For this review, take the finished solid that the model builds, in its own axes (mm). A direction names the side the tool comes from. Round coordinates to 2 decimals unless told otherwise and drop trailing zeros. Order: outer loops, then holes, each group sorted by start corner. A loop starts at its lowest first (then second) coordinate and runs counter-clockwise, first axis right, second up.
from build123d import *

# Parameters (mm, degrees)
F1_DEPTH = 25.4


with BuildPart() as f1:
    # F0 (on Front) → F1 (new body)
    with BuildSketch(Plane.XZ):
        with BuildLine():
            Line((-59.0061545372, 19.8315382004), (-59.0061545372, 0))
            Line((-59.0061545372, 0), (-57.6384626329, 0))
            Line((-57.6384626329, 0), (-52.8619785953, 0))
            ThreePointArc((-52.8619785953, 0), (-52.785725887, 1.0863777847), (-52.5584630668, 2.1514518559))
            Line((-52.5584630668, 2.1514518559), (-52.5584630668, 5.3730774671))
            Line((-52.5584630668, 5.3730774671), (-48.7484624609, 9.183078073))
            Line((-48.7484624609, 9.183078073), (-41.4215400815, 9.183078073))
            Line((-41.4215400815, 9.183078073), (-37.6115394756, 5.3730774671))
            Line((-37.6115394756, 5.3730774671), (-37.6115394756, 4.7639395972))
            ThreePointArc((-37.6115394756, 4.7639395972), (-38.2208958426, 4.7248074356), (-38.8202414059, 4.6080538331))
            ThreePointArc((-38.8202414059, 4.6080538331), (-37.6957431315, 2.4249207086), (-37.3080239472, 0))
            Line((-37.3080239472, 0), (23.1979270853, 0))
            ThreePointArc((23.1979270853, 0), (23.2602248919, 1.000404867), (23.446155712, 1.9853518934))
            ThreePointArc((23.446155712, 1.9853518934), (30.0178470159, 7.9671258273), (38.0999986082, 4.2728638401))
            ThreePointArc((38.0999986082, 4.2728638401), (39.0128166681, 2.2225195794), (39.3251548134, 0))
            Line((39.3251548134, 0), (48.2600033283, 0))
            Line((48.2600033283, 0), (48.2600033283, 16.9007703662))
            Line((48.2600033283, 16.9007703662), (48.2600033283, 19.8315382004))
            Line((48.2600033283, 19.8315382004), (47.6738475263, 22.3715398461))
            Line((47.6738475263, 22.3715398461), (25.399999693, 22.3715398461))
            Line((25.399999693, 22.3715398461), (12.1138468385, 35.6576927006))
            Line((12.1138468385, 35.6576927006), (-28.3307693899, 35.6576927006))
            Line((-28.3307693899, 35.6576927006), (-28.3307693899, 19.8315382004))
            Line((-28.3307693899, 19.8315382004), (-59.0061545372, 19.8315382004))
        make_face()
        with BuildLine():
            ThreePointArc((-52.5584630668, 2.1514518559), (-52.785725887, 1.0863777847), (-52.8619785953, 0))
            Line((-52.8619785953, 0), (-52.5584630668, 0))
            Line((-52.5584630668, 0), (-52.5584630668, 2.1514518559))
        make_face()
        with BuildLine():
            Line((-52.5584630668, 0), (-52.8619785953, 0))
            ThreePointArc((-52.8619785953, 0), (-45.0850012712, -7.776977324), (-37.3080239472, 0))
            ThreePointArc((-37.3080239472, 0), (-37.6957431315, 2.4249207086), (-38.8202414059, 4.6080538331))
            ThreePointArc((-38.8202414059, 4.6080538331), (-46.4539291026, 7.6555478505), (-52.5584630668, 2.1514518559))
            Line((-52.5584630668, 2.1514518559), (-52.5584630668, 0))
        make_face()
        with BuildLine():
            Line((23.446155712, 0), (23.1979270853, 0))
            ThreePointArc((23.1979270853, 0), (31.2615409493, -8.0636138641), (39.3251548134, 0))
            Line((39.3251548134, 0), (38.0999986082, 0))
            Line((38.0999986082, 0), (23.446155712, 0))
        make_face()
        with BuildLine():
            ThreePointArc((23.446155712, 1.9853518934), (23.2602248919, 1.000404867), (23.1979270853, 0))
            Line((23.1979270853, 0), (23.446155712, 0))
            Line((23.446155712, 0), (23.446155712, 1.9853518934))
        make_face()
        with BuildLine():
            Line((38.0999986082, 0), (39.3251548134, 0))
            ThreePointArc((39.3251548134, 0), (39.0128166681, 2.2225195794), (38.0999986082, 4.2728638401))
            Line((38.0999986082, 4.2728638401), (38.0999986082, 0))
        make_face()
        with BuildLine():
            ThreePointArc((38.0999986082, 4.2728638401), (30.0178470159, 7.9671258273), (23.446155712, 1.9853518934))
            Line((23.446155712, 1.9853518934), (23.446155712, 0))
            Line((23.446155712, 0), (38.0999986082, 0))
            Line((38.0999986082, 0), (38.0999986082, 4.2728638401))
        make_face()
    extrude(amount=F1_DEPTH)


solid = f1.part
(1) Add section A-A on y = -23. Give the boundary of the cut face in (x, z) (3 decimals).
(2) Wall thickness on L1, parallel to X at y = -18.75, z = 6; L2, parallel to X at y = -21.75, z = -0.5; L3, parallel to X at y = -1.5, z = -6: over which ranges is each line inside the solid? List them lowest first.
(3) Draft analysis for pull direction Z (two halves, no side actions). For faces 6 (the face through (-28.331, -13, 28)), 7 (the face through (-50.68, -12.52, 7.25)), 8 (the face through (-8, -13, 35.658)), 9 (the face through (-46.334, -12.522, 7.676)), state which applies: pulls with the +Z half, pulls with the -Z half, needs draft (parallel to the pull), parting line crosses it, or undercut.
(4) Add section C-C on z = 30. Give the boundary of the cut face in (x, y), plus the area to 3 significant figures.
(5) Add section B-B on x = -33. Give the boundary of the cut face in (y, z).
(6) Tool access review of faces 1 (the face through (44, -13, 0)), 2 (the face through (37, -13, 22.372)), 3 (the face through (-56, -13, 0)), 4 (the face through (-7, -13, 0)), 5 (the face through (-45, -13, 9.183)): name each direction out of +Z, -Z, +X, -X, +Y, -Y from which nothing blocks a thin tool from reaching the whole face with its end or side.
(7) Clearance check with flat-ended pins moving along their axes: P1, Ø7, axis at x = -57, y = -12, coming from the -Z side; P2, Ø6, axis at y = -12.5, z = 26.5, coming from the +X side; P3, Ø8, axis at x = 24, y = -15.5, coming from the +Z side. State where each tip first meets the part, or that it passes through.
Here are the results:
1. outline: (-59.006, 0) - (-52.862, 0) arc R7.777 ccw to (-37.308, 0) - (23.198, 0) arc R8.064 ccw to (39.325, 0) - (48.26, 0) - (48.26, 19.832) - (47.674, 22.372) - (25.4, 22.372) - (12.114, 35.658) - (-28.331, 35.658) - (-28.331, 19.832) - (-59.006, 19.832) - close; hole (-52.558, 2.151) arc R7.777 cw to (-38.82, 4.608) arc R4.764 cw to (-37.612, 4.764) - (-37.612, 5.373) - (-41.422, 9.183) - (-48.748, 9.183) - (-52.558, 5.373) - close
2. L1: x = -59.01 to -51.93, -50.03 to -40.14, -38.24 to 48.26
2. L2: x = -52.85 to -37.32, 23.21 to 39.31
2. L3: x = -50.03 to -40.14, 25.87 to 36.65
3. face 6: needs draft
3. face 7: undercut
3. face 8: pulls with the +Z half
3. face 9: undercut
4. outline: (-28.33, -25.4) - (17.77, -25.4) - (17.77, 0) - (-28.33, 0) - close
4. area: 1,170 mm2
5. outline: (-25.4, 0) - (0, 0) - (0, 19.83) - (-25.4, 19.83) - close
6. face 1: -Z, +X, +Y, -Y
6. face 2: +Z, +X, +Y, -Y
6. face 3: -Z, -X, +Y, -Y
6. face 4: -Z, +Y, -Y
6. face 5: +Y, -Y
7. P1: stops at z = 0
7. P2: stops at x = 24.27
7. P3: stops at z = 27.77
